```python
from build123d import *

# Parameters (mm, degrees)
F1_DEPTH       = 30
F2_R           = 0.2
F3_R           = 2
F5_DEPTH       = 10
F8_DEPTH       = 6
F8_DEPTH_BACK  = 10
F10_DEPTH      = 12
F11_R          = 5
F12_DEPTH      = 40.4696358235
F12_DEPTH_BACK = 16.8323643765
F13_R          = 2
F14_R          = 5


# Not quite as in the source:
# - ends of sketch curves that miss each other by under 0.0002 mm in the source are joined


with BuildPart() as f1:
    # F0 (on Top) → F1 (new body)
    with BuildSketch(Plane.XY):
        with BuildLine():
            ThreePointArc((-4.2249260349, 0.8), (-1.4496004126, 4.0482908299), (2.7568097504, 3.3))
            Line((2.7568097504, 3.3), (5.7568097504, 6.3))
            Line((5.7568097504, 6.3), (0, 6.3))
            add(Edge.make_bspline(
                [(0, 6.3), (-4.1648952214, 6.3), (-17.5449881237, 1.3096127619), (-2.8048020259, -10.5313642765), (0, -10.5313642765)],
                knots=[0, 0, 0, 0, 0.475816506, 1, 1, 1, 1], degree=3))
            Line((0, -10.5313642765), (42.8038475773, -10.5313642765))
            Line((42.8038475773, -10.5313642765), (62.1961524227, -10.5313642765))
            Line((62.1961524227, -10.5313642765), (70, -10.5313642765))
            add(Edge.make_bspline(
                [(76.8431902496, 0), (76.8431902496, -2.967218801), (74.0984288633, -10.5313642765), (70, -10.5313642765)],
                knots=[0, 0, 0, 0, 0.4787052711, 0.4787052711, 0.4787052711, 0.4787052711], degree=3))
            Line((76.8431902496, 0), (76.8431902496, 6.3))
            Line((76.8431902496, 6.3), (73.3, 2.7568097504))
            ThreePointArc((73.3, 2.7568097504), (74.0422765863, 1.4662878299), (74.3, 0))
            ThreePointArc((74.3, 0), (73.311344138, -2.7431733449), (70.8, -4.2249260349))
            ThreePointArc((70.8, -4.2249260349), (71.4937369246, -4.86963515), (71.75, -5.7813642765))
            ThreePointArc((71.75, -5.7813642765), (69.0882708736, -7.2751012011), (69.2, -4.2249260349))
            ThreePointArc((69.2, -4.2249260349), (65.9517091701, -1.4496004126), (66.7, 2.7568097504))
            Line((66.7, 2.7568097504), (63.1568097504, 6.3))
            Line((63.1568097504, 6.3), (59.5214758241, 6.3))
            Line((59.5214758241, 6.3), (57, -8))
            Line((57, -8), (48, -8))
            Line((48, -8), (46.5893841543, 0))
            Line((46.5893841543, 0), (11.889675867, 0))
            Line((11.889675867, 0), (8.7784060298, -3.1112698372))
            ThreePointArc((8.7784060298, -3.1112698372), (5.8049742519, -4.3978404552), (2.7568097504, -3.3))
            ThreePointArc((2.7568097504, -3.3), (-1.4496004126, -4.0482908299), (-4.2249260349, -0.8))
            ThreePointArc((-4.2249260349, -0.8), (-7.5313642765, 0), (-4.2249260349, 0.8))
        make_face()
        Polygon((62.1961524227, -10.5313642765), (42.8038475773, -10.5313642765), (48, -13.5313642765), (57, -13.5313642765), align=None)
    extrude(amount=F1_DEPTH)

    # F2
    f2_edges = [f1.edges().sort_by_distance(p)[0] for p in [
        (5.75681, 6.3, 15),
        (2.75681, 3.3, 15),
        (-4.224926, 0.8, 15),
        (-4.224926, -0.8, 15),
        (2.75681, -3.3, 15),
        (76.84319, 6.3, 15),
        (66.7, 2.75681, 15),
        (69.2, -4.224926, 15),
        (70.8, -4.224926, 15),
        (73.3, 2.75681, 15),
    ]]
    fillet(f2_edges, radius=F2_R)

    # F3
    f3_edges = [f1.edges().sort_by_distance(p)[0] for p in [
        (63.15681, 6.3, 15),
        (48, -8, 15),
        (59.521476, 6.3, 15),
        (46.589384, 0, 15),
        (57, -8, 15),
        (11.889676, 0, 15),
        (42.803848, -10.531364, 15),
        (48, -13.531364, 15),
        (57, -13.531364, 15),
        (62.196152, -10.531364, 15),
    ]]
    fillet(f3_edges, radius=F3_R)

    # F4 (on face) → F5 (join)
    with BuildSketch(Plane(origin=(0, 0, 0), x_dir=(1, 0, 0), z_dir=(0, 0, -1))):
        with BuildLine():
            Line((28.5358983849, 51), (28.5358983849, 10.5313642765))
            Line((28.5358983849, 10.5313642765), (42.2679491924, 10.5313642765))
            ThreePointArc((42.2679491924, 10.5313642765), (42.7855872826, 10.5995126239), (43.2679491924, 10.7993134689))
            Line((43.2679491924, 10.7993134689), (47.5358983849, 13.2634150841))
            ThreePointArc((47.5358983849, 13.2634150841), (48.0182602947, 13.4632159291), (48.5358983849, 13.5313642765))
            Line((48.5358983849, 13.5313642765), (48.5358983849, 51))
            Line((48.5358983849, 51), (28.5358983849, 51))
        make_face()
        with BuildLine():
            ThreePointArc((35.5358983849, 40.5313642765), (40.5358983849, 45.5313642765), (45.5358983849, 40.5313642765))
            Line((45.5358983849, 40.5313642765), (45.5358983849, 25.5313642765))
            ThreePointArc((45.5358983849, 25.5313642765), (40.5358983849, 20.5313642765), (35.5358983849, 25.5313642765))
            Line((35.5358983849, 25.5313642765), (35.5358983849, 40.5313642765))
        make_face(mode=Mode.SUBTRACT)
    extrude(amount=-F5_DEPTH)

    # F7 (on offset) → F8 (join, two sides)
    with BuildSketch(Plane(origin=(18.5358983849, 0, 0), x_dir=(0, -1, 0), z_dir=(-1, 0, 0))) as f8_sk:
        with BuildLine():
            ThreePointArc((14.8303992429, 0), (11.0259152701, 15.1935946786), (16.1337307537, 30))
            Line((16.1337307537, 30), (10.5313622104, 30))
            Line((10.5313622104, 30), (10.5313642765, 0))
            Line((10.5313642765, 0), (14.8303992429, 0))
        make_face()
    extrude(amount=F8_DEPTH)
    extrude(f8_sk.sketch, amount=-F8_DEPTH_BACK)

    # F9 (on face) → F10 (cut)
    with BuildSketch(Plane(origin=(12.5358983849, 0, 0), x_dir=(0, -1, 0), z_dir=(-1, 0, 0))):
        with BuildLine():
            Line((10.5313642765, 0.6300555063), (10.5313642765, 27.3699444937))
            ThreePointArc((10.5313642765, 27.3699444937), (7.5, 14), (10.5313642765, 0.6300555063))
        make_face()
    extrude(amount=F10_DEPTH, mode=Mode.SUBTRACT)

    # F11 (on face) → F12 (cut, two sides)
    with BuildSketch(Plane.XZ.offset(10.5313642765)) as f12_sk:
        with Locations((18.5358983849, 14)):
            Circle(F11_R)
    extrude(amount=F12_DEPTH, mode=Mode.SUBTRACT)
    extrude(f12_sk.sketch, amount=-F12_DEPTH_BACK, mode=Mode.SUBTRACT)

    # F13
    f13_edges = [f1.edges().sort_by_distance(p)[0] for p in [
        (48.535898, -13.531364, 5),
        (48.535898, -13.531364, 20),
    ]]
    fillet(f13_edges, radius=F13_R)

    # F14
    f14_edges = [f1.edges().sort_by_distance(p)[0] for p in [
        (28.535898, -51, 5),
        (48.535898, -51, 5),
    ]]
    fillet(f14_edges, radius=F14_R)


solid = f1.part
```
Can you work these out from the model? Positions are in its coordinate system, mm. A direction names the side the tool comes from. Round coordinates to 2 decimals unless told otherwise and drop trailing zeros. Loops run counter-clockwise (first coordinate to the right, second up) from the corner with the lowest first, then second, coordinate; pieces in that order, holes last. Notation, with made-up numbers: M 39.5,70 L 95.5,70 A22 ccw 95.5,97 Z; hole C -3.5,60.25 d5. An arc over 180 degrees is marked long. Answer as a JSON object with one key per item and string values. Group by question number.
Q1. On a 3-axis mill with a long thin cutter (end or side, diameter ignored), from which of +Z, -Z, +X, -X, +Y, -Y can I reach the whole of each face in a straight line? I mean faces 4 (the flat face through (65.178, 4.279, 14.79)), 5 (the flat face through (45.372, -12.014, 19.86)), 6 (the cylindrical face through (6.6, -7.5, 14.2)), 7 (the flat face through (66, -10.531, 15)), 8 (the cylindrical face through (40.646, -20.533, 4.93)). Say none if no direction works.
Q2. Will these pins go through, and if not, where does the flat tip stop? pin 1 (1.7 mm diameter, centred on x = 53, z = 20, fed in from +Y); pin 2 (6 mm diameter, centred on x = 18.54, z = 14, fed in from +Y); pin 3 (3 mm diameter, centred on y = -33.5, z = 7.5, fed in from -X); pin 4 (8.5 mm diameter, centred on x = 51.5, z = 7.5, fed in from -Y).
Q3. Imagine slicing it at A-A, the plane y = -30. Please give me the cut outline in (x, z), then the cut area to 3 significant figures.
Q4. Imagine slicing it at B-B, the plane y = -9.5. Count the separate pieces of the cut face and the enclosed holes in it, then the cut area to 3 significant figures.
Q5. Please list where these lines run through material, in increasing order: L1, parallel to X at y = -28, z = 3.5; L2, parallel to X at y = 4.5, z = 16; L3, parallel to Y at x = 5, z = 5.5.
Q6. We'd pull the mould along Y, two halves only. Please class faces 1 (the cylindrical face through (47.11, -49.496, 5.07)), 2 (the flat face through (45.536, -33, 5)), 3 (the cylindrical face through (56.592, -7.545, 15.21)): +Y half, -Y half, draft (parallel to the pull), parting line (faces both ways), or undercut.
Findings:
{
 "1": {"face 4": "+Z, -Z, +Y", "face 5": "+Z, -Y", "face 6": "-Y", "face 7": "+Z, -Z, +X, -Y", "face 8": "+Z, -Z"},
 "2": {"pin 1": "stops at y = -8", "pin 2": "passes through", "pin 3": "stops at x = 28.54", "pin 4": "stops at y = -49.35"},
 "3": {"outline": "M 28.54,0 L 35.54,0 L 35.54,10 L 28.54,10 Z; M 45.54,0 L 48.54,0 L 48.54,10 L 45.54,10 Z", "area": "100 mm2"},
 "4": {"separate pieces": "1", "enclosed holes": "2", "area": "1,920 mm2"},
 "5": {"L1": "x = 28.54 to 35.54, 45.54 to 48.54", "L2": "x = -7.06 to 3.96, 59.2 to 64.96, 75.04 to 76.84", "L3": "y = -8.69 to -4.35, 5.54 to 6.3"},
 "6": {"face 1": "-Y half", "face 2": "undercut", "face 3": "+Y half"}
}
